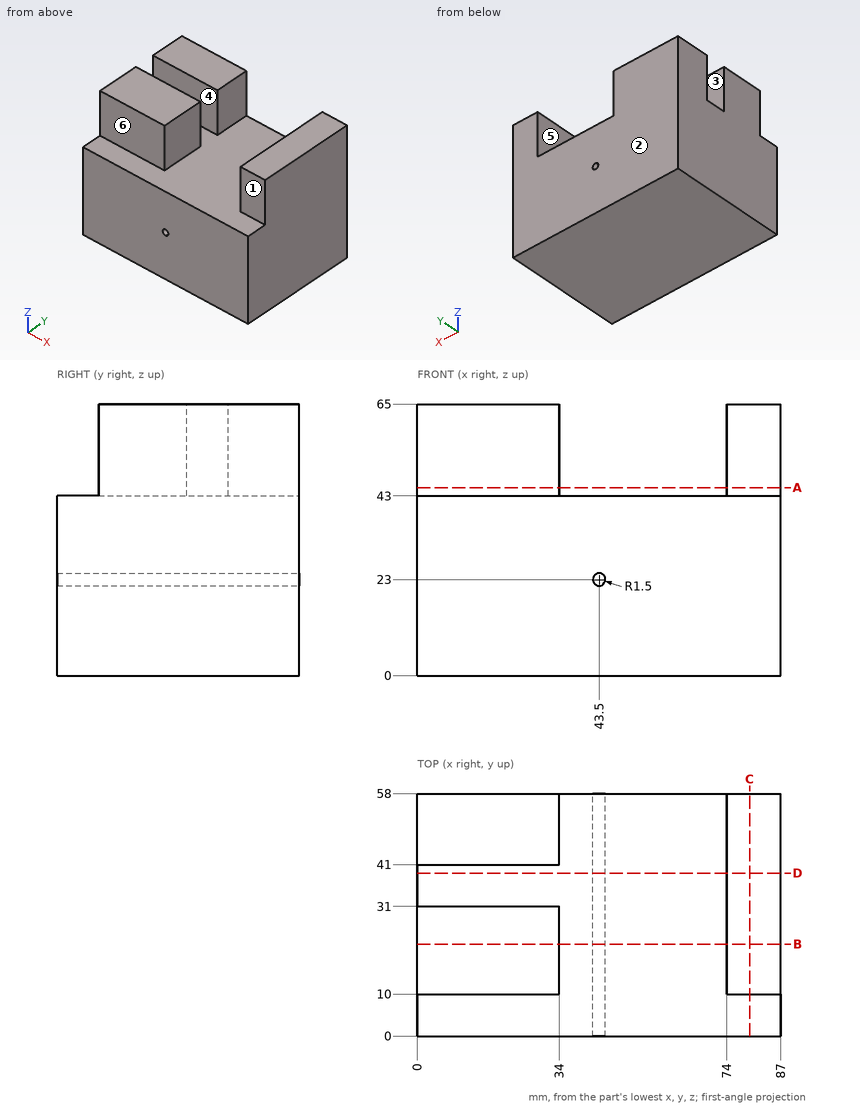
Job drawing, mm, ordinate dimensions from the low corner. One solid piece. A direction names the side the tool comes from. Give positions to 0.01 mm unless a question says otherwise; leave off trailing zeros. Loops run counter-clockwise (first coordinate to the right, second up) from the corner with the lowest first, then second, coordinate; pieces in that order, holes last. Notation, with made-up numbers: M -12,7 L 15,7 A13 cw 15,29 Z; hole C -29,26 d5. An arc over 180 degrees is marked long. Answer in a Markdown table with one row per item. Add a question column.
Item 1: Band-saw the part on B-B on y = 22. Give the cut face in (x, z), then the cut area to 3 significant figures.
Item 2: Mould opens along Y. For the marked faces 1, 2 and 3 say: +Y half, -Y half, draft (parallel to the pull), parting line (faces both ways), or undercut.
Item 3: Tool access for the marked faces 4, 5 and 6: list every direction of +Z, -Z, +X, -X, +Y, -Y with a clear straight run to the whole face (end or side of a thin tool).
Item 4: Band-saw the part on C-C on x = 79.5. Give the cut face in (y, z).
Item 5: Probe probe 1 along X at (y, z) = (20.5, 53); probe 2 along Y at (x, z) = (28, 58.5); probe 3 along Z at (x, y) = (52, 47). List the from-to ranges inside material, lowest first.
Item 6: Band-saw the part on A-A on z = 45. Give the cut face in (x, y), then the cut area to 3 significant figures.
Item 7: Band-saw the part on D-D on y = 39. Give the cut face in (x, z).
Item 8: Drop flat-ended pins along their axis: P1, Ø8, axis at x = 61, y = 38.5, coming from the +Z side; P2, Ø6.5, axis at x = 18.5, z = 50.5, coming from the -Y side. Give the stop position or say it passes through.
Reply:
| question | item | result |
|---|---|---|
| 1 | outline | M 0,0 L 87,0 L 87,65 L 74,65 L 74,43 L 34,43 L 34,65 L 0,65 Z; hole C 43.5,23 d3 |
| 1 | area | 4,770 mm^2 |
| 2 | face 1 | -Y half |
| 2 | face 2 | +Y half |
| 2 | face 3 | undercut |
| 3 | face 4 | +Z, -X |
| 3 | face 5 | +Z, +Y, -Y |
| 3 | face 6 | +Z, +X, -X, -Y |
| 4 | outline | M 0,0 L 58,0 L 58,65 L 10,65 L 10,43 L 0,43 Z |
| 5 | probe 1 | x = 0 to 34, 74 to 87 |
| 5 | probe 2 | y = 10 to 31, 41 to 58 |
| 5 | probe 3 | z = 0 to 43 |
| 6 | outline | M 0,10 L 34,10 L 34,31 L 0,31 Z; M 0,41 L 34,41 L 34,58 L 0,58 Z; M 74,10 L 87,10 L 87,58 L 74,58 Z |
| 6 | area | 1,920 mm^2 |
| 7 | outline | M 0,0 L 87,0 L 87,65 L 74,65 L 74,43 L 0,43 Z; hole C 43.5,23 d3 |
| 8 | P1 | stops at z = 43 |
| 8 | P2 | stops at y = 10 |
